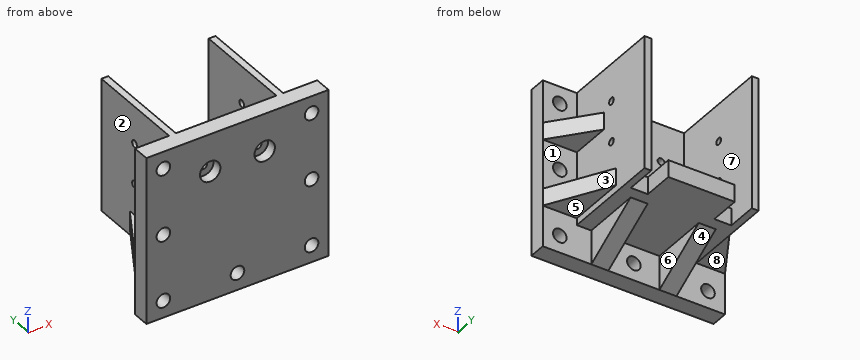
```python
from build123d import *

# Parameters (mm, degrees)
ESQUISSE1_W             = 33.5
ESQUISSE1_H             = 39
BOSS_EXTRU_1_DEPTH      = 49
ESQUISSE3_W             = 29.5
ESQUISSE3_H             = 44
ENL_V_MAT_EXTRU_1_DEPTH = 34
ESQUISSE4_W             = 53.5
ESQUISSE4_H             = 49
BOSS_EXTRU_2_DEPTH      = 5
ESQUISSE5_R             = 2
ENL_V_MAT_EXTRU_2_DEPTH = 5
NERVURE3_REACH          = 67.365
ESQUISSE8_WALL_W        = 148.286921202
ESQUISSE8_WALL_H        = 5
NERVURE4_REACH          = 67.626
ESQUISSE9_WALL_W        = 153.252619022
ESQUISSE9_WALL_H        = 5
NERVURE5_REACH          = 69.984
ESQUISSE10_WALL_W       = 157.967827076
ESQUISSE10_WALL_H       = 5
ESQUISSE11_R            = 1.025
ENL_V_MAT_EXTRU_3_DEPTH = 5
ESQUISSE13_W            = 39
ESQUISSE13_H            = 14.190780958
ENL_V_MAT_EXTRU_5_DEPTH = 72.857497869
SYM_TRIE6_START         = 25.809219042
SYM_TRIE6_OUTLINE_W     = 5
SYM_TRIE6_OUTLINE_H     = 5
SYM_TRIE6_DEPTH         = 9
SYM_TRIE6_2_OUTLINE_R   = 3
SYM_TRIE6_2_DEPTH       = 3
SYM_TRIE6_START_2       = 3
SYM_TRIE6_3_OUTLINE_R   = 1.025
SYM_TRIE6_3_DEPTH       = 2


# Read off the part's stored shape, not the designer's step: Symétrie6
with BuildPart() as part:
    # Esquisse1 → Boss.-Extru.1 (new body)
    with BuildSketch(Plane(origin=(0, 0, 0), x_dir=(1, 0, 0), z_dir=(0, 1, 0))):
        Rectangle(ESQUISSE1_W, ESQUISSE1_H)
    extrude(amount=BOSS_EXTRU_1_DEPTH)

    # Esquisse3 → Enlèv. mat.-Extru.1 (cut)
    with BuildSketch(Plane.XY.offset(19.5)):
        with Locations((0, 27)):
            Rectangle(ESQUISSE3_W, ESQUISSE3_H)
    extrude(amount=-ENL_V_MAT_EXTRU_1_DEPTH, mode=Mode.SUBTRACT)

    # Esquisse4 → Boss.-Extru.2 (add)
    with BuildSketch(Plane(origin=(0, 0, 0), x_dir=(1, 0, 0), z_dir=(0, 1, 0))):
        with Locations((0, 5)):
            Rectangle(ESQUISSE4_W, ESQUISSE4_H)
    extrude(amount=BOSS_EXTRU_2_DEPTH)

    # Esquisse5 → Enlèv. mat.-Extru.2 (cut)
    with BuildSketch(Plane(origin=(0, 5, 0), x_dir=(1, 0, 0), z_dir=(0, 1, 0))):
        with Locations(Location((-21.75, 24.5, 0), (0, 0, 270))):
            Circle(ESQUISSE5_R)
        with Locations(Location((0, 24.5, 0), (0, 0, 270))):
            Circle(ESQUISSE5_R)
        with Locations(Location((21.75, 24.5, 0), (0, 0, 270))):
            Circle(ESQUISSE5_R)
        with Locations(Location((21.75, 5, 0), (0, 0, 270))):
            Circle(ESQUISSE5_R)
        with Locations(Location((21.75, -14.5, 0), (0, 0, 270))):
            Circle(ESQUISSE5_R)
        with Locations(Location((-21.75, -14.5, 0), (0, 0, 270))):
            Circle(ESQUISSE5_R)
        with Locations(Location((-21.75, 5, 0), (0, 0, 270))):
            Circle(ESQUISSE5_R)
    extrude(amount=-ENL_V_MAT_EXTRU_2_DEPTH, mode=Mode.SUBTRACT)

    # Esquisse8 wall → Nervure3 (add, up to next)
    with BuildSketch(Plane(origin=(21.75, 10.958767963, 4.5), x_dir=(-0.642787609685, 0.766044443121, 0), z_dir=(-0.766044443121, -0.642787609685, 0)), mode=Mode.PRIVATE) as nervure3_sk1:
        Rectangle(ESQUISSE8_WALL_W, ESQUISSE8_WALL_H)
    nervure3_tool1 = extrude(nervure3_sk1.sketch, amount=NERVURE3_REACH, mode=Mode.PRIVATE) - part.part
    nervure3 = nervure3_tool1.solids().sort_by_distance((21.75, 10.958767963, 4.5))[0]
    add(nervure3)

    # Esquisse9 wall → Nervure4 (add, up to next)
    with BuildSketch(Plane(origin=(21.75, 13.660254038, -15), x_dir=(-0.499999999993, 0.866025403788, 0), z_dir=(-0.866025403788, -0.499999999993, 0)), mode=Mode.PRIVATE) as nervure4_sk1:
        Rectangle(ESQUISSE9_WALL_W, ESQUISSE9_WALL_H)
    nervure4_tool1 = extrude(nervure4_sk1.sketch, amount=NERVURE4_REACH, mode=Mode.PRIVATE) - part.part
    nervure4 = nervure4_tool1.solids().sort_by_distance((21.75, 13.660254038, -15))[0]
    add(nervure4)

    # Esquisse10 wall → Nervure5 (add, up to next)
    with BuildSketch(Plane(origin=(10, 13.660254038, -24.5), x_dir=(0, 0.866025403788, 0.499999999993), z_dir=(0, -0.499999999993, 0.866025403788)), mode=Mode.PRIVATE) as nervure5_sk1:
        Rectangle(ESQUISSE10_WALL_W, ESQUISSE10_WALL_H)
    nervure5_tool1 = extrude(nervure5_sk1.sketch, amount=NERVURE5_REACH, mode=Mode.PRIVATE) - part.part
    nervure5 = nervure5_tool1.solids().sort_by_distance((10, 13.660254038, -24.5))[0]
    add(nervure5)

    # Symétrie1: Nervure5 across plane
    add(nervure5.mirror(Plane(origin=(0, 0, 0), x_dir=(0, 0, 1), z_dir=(1, 0, 0))))

    # Symétrie3: Nervure3, Nervure4 across plane
    add(nervure3.mirror(Plane(origin=(0, 0, 0), x_dir=(0, 0, 1), z_dir=(1, 0, 0))))
    add(nervure4.mirror(Plane(origin=(0, 0, 0), x_dir=(0, 0, 1), z_dir=(1, 0, 0))))

    # Esquisse11 → Enlèv. mat.-Extru.3 (cut)
    with BuildSketch(Plane.ZY.offset(16.75)):
        with Locations((-3.5, 44.25)):
            Circle(ESQUISSE11_R)
        with Locations((8.5, 44.25)):
            Circle(ESQUISSE11_R)
        with Locations((-3.5, 20.25)):
            Circle(ESQUISSE11_R)
        with Locations((8.5, 20.25)):
            Circle(ESQUISSE11_R)
    enl_v_mat_extru_3 = extrude(amount=-ENL_V_MAT_EXTRU_3_DEPTH, mode=Mode.SUBTRACT)

    # Symétrie4: Enlèv. mat.-Extru.3 across plane
    add(enl_v_mat_extru_3.mirror(Plane(origin=(0, 0, 0), x_dir=(0, 0, 1), z_dir=(1, 0, 0))), mode=Mode.SUBTRACT)

    # Esquisse13 → Enlèv. mat.-Extru.5 (cut, through all)
    with BuildSketch(Plane(origin=(16.75, 0, 0), x_dir=(0, 0, -1), z_dir=(1, 0, 0))):
        with Locations((0, 41.904609521)):
            Rectangle(ESQUISSE13_W, ESQUISSE13_H)
    extrude(amount=-ENL_V_MAT_EXTRU_5_DEPTH, mode=Mode.SUBTRACT)

    # Symétrie6 outline → Symétrie6 (cut)
    with BuildSketch(Plane(origin=(0, 0, 0), x_dir=(1, 0, 0), z_dir=(0, 1, 0)).offset(SYM_TRIE6_START)):
        with Locations((-12.25, 17)):
            Rectangle(SYM_TRIE6_OUTLINE_W, SYM_TRIE6_OUTLINE_H)
        with Locations((12.25, 17)):
            Rectangle(SYM_TRIE6_OUTLINE_W, SYM_TRIE6_OUTLINE_H)
    extrude(amount=SYM_TRIE6_DEPTH, mode=Mode.SUBTRACT)

    # Sym_trie6 2 outline → Sym_trie6 2 (cut)
    with BuildSketch(Plane(origin=(0, 0, 0), x_dir=(1, 0, 0), z_dir=(0, 1, 0))):
        with Locations((8, -8.5)):
            Circle(SYM_TRIE6_2_OUTLINE_R)
        with Locations((-8, -8.5)):
            Circle(SYM_TRIE6_2_OUTLINE_R)
    extrude(amount=SYM_TRIE6_2_DEPTH, mode=Mode.SUBTRACT)

    # Sym_trie6 3 outline → Sym_trie6 3 (cut)
    with BuildSketch(Plane(origin=(0, 0, 0), x_dir=(1, 0, 0), z_dir=(0, 1, 0)).offset(SYM_TRIE6_START_2)):
        with Locations((8, -8.5)):
            Circle(SYM_TRIE6_3_OUTLINE_R)
        with Locations((-8, -8.5)):
            Circle(SYM_TRIE6_3_OUTLINE_R)
    extrude(amount=SYM_TRIE6_3_DEPTH, mode=Mode.SUBTRACT)


solid = part.part
```
The listing builds one solid part. Answer for the finished solid, in the listing's coordinates (mm). Face numbers are marked on the shaded views. A direction names the side the tool comes from. Coordinates: 2 decimals unless noted, no trailing zeros. Write each loop counter-clockwise with the first axis right and the second up, starting at its lowest first coordinate (ties: lowest second). Pieces come first, ordered by that corner, then holes. Notation, with made-up numbers: (33.5, 20) - (85.5, 20) arc R28 cw to (85.5, 57) - close; hole circle Ø9 at (-28, -14). An arc over 180 degrees is marked (long way). One line per item, written item: value.
1) For a pull along Z with two mould halves and no side action, classify the marked faces 1, 2, 3 and 4 as pulls with the +Z half, pulls with the -Z half, needs draft (parallel to the pull), parting line crosses it, or undercut.
Geometry check:
face 1: undercut
face 2: undercut
face 3: needs draft
face 4: pulls with the -Z half
2) A tool of negligible diameter and unlimited length cuts with its end or side. For the marked faces 5, 6, 7 and 8, from which of +Z, -Z, +X, -X, +Y, -Y can it reach the whole face along a straight path? Write none if from no direction.
Geometry check:
face 5: -Z, +X, +Y
face 6: -Z, +Y
face 7: +Z, +Y
face 8: -Z, -X, +Y
3) Each of these flat-tipped pins is pushed along its axis until it touches: pin 1 Ø5 at (y, z) = (31.5, 4.5) entering from -X; pin 2 Ø3 at (x, z) = (21, -6) entering from +Y; pin 3 Ø1.8 at (y, z) = (20.25, -3.5) entering from -X; pin 4 Ø8 at (x, y) = (21.5, 11) entering from -Z. Where does it stop, or does it pass through?
Geometry check:
pin 1: stops at x = -16.75
pin 2: stops at y = 5
pin 3: passes through
pin 4: stops at z = -17.5
4) Find section B-B (y = 32). Give the vertices of the cut face in (x, z), and give its area (4 significant figures).
Geometry check:
outline: (-16.75, -19.5) - (-14.75, -19.5) - (-14.75, 19.5) - (-16.75, 19.5) - close; (-9.75, -19.5) - (9.75, -19.5) - (9.75, -14.5) - (-9.75, -14.5) - close; (14.75, -19.5) - (16.75, -19.5) - (16.75, 19.5) - (14.75, 19.5) - close
area: 253.5 mm2
5) Find section A-A (x = 0). Give the vertices of the cut face in (y, z), and give its area (3 significant figures).
Geometry check:
outline: (0, -29.5) - (5, -29.5) - (5, -26.5) - (0, -26.5) - close; (0, -22.5) - (5, -22.5) - (5, -19.5) - (34.81, -19.5) - (34.81, -14.5) - (5, -14.5) - (5, 19.5) - (0, 19.5) - close
area: 374 mm2
6) Consider line 1 along X through (y, z) = (3.5, 14.5); line 2 along Z through (x, y) = (16.35, 20.25) (3 decimals); line 3 along X through (y, z) = (1.75, -24.5). Determine where each line is inside the solid, lowest interval first. Write a range as from..to.
Geometry check:
line 1: x = -26.75..-23.75, -19.75..19.75, 23.75..26.75
line 2: z = -19.5..-4.525, -2.475..7.475, 9.525..19.5
line 3: x = -26.75..-23.75, -19.75..-2, 2..19.75, 23.75..26.75
7) Find section C-C (z = -24.5). Give the vertices of the cut face in (x, y).
Geometry check:
outline: (-26.75, 0) - (-23.75, 0) - (-23.75, 5) - (-26.75, 5) - close; (-19.75, 0) - (-2, 0) - (-2, 5) - (-7.5, 5) - (-7.5, 13.66) - (-12.5, 13.66) - (-12.5, 5) - (-19.75, 5) - close; (2, 0) - (19.75, 0) - (19.75, 5) - (12.5, 5) - (12.5, 13.66) - (7.5, 13.66) - (7.5, 5) - (2, 5) - close; (23.75, 0) - (26.75, 0) - (26.75, 5) - (23.75, 5) - close
8) Find section D-D (x = -16). Give the vertices of the cut face in (y, z) (3 decimals), and give its area (3 significant figures).
Geometry check:
outline: (0, -29.5) - (5, -29.5) - (5, -19.5) - (34.809, -19.5) - (34.809, 19.5) - (0, 19.5) - close; hole circle Ø2.05 at (20.25, -3.5); hole circle Ø2.05 at (20.25, 8.5)
area: 1,400 mm2
